Read the model definition and answer for the solid it produces. Units are mm, in the model's axes. A direction names the side the tool comes from. Coordinates: 2 decimals unless noted, no trailing zeros. Order: outer loops, then holes, each group sorted by start corner. A loop starts at its lowest first (then second) coordinate and runs counter-clockwise, first axis right, second up. Notation, with made-up numbers: M -25.5,65 L -3.5,65 A19 ccw -3.5,84 Z; hole C 28,6.25 d11. An arc over 180 degrees is marked long. Use a Markdown table: item, result. Add a question column.
1) Each of these flat-tipped pins is pushed along its axis until it touches: pin 1 Ø3.5 at (x, y) = (8, -20.16) entering from -Z; pin 2 Ø1 at (x, y) = (0.5, -19) entering from +Z; pin 3 Ø4 at (y, z) = (-3.5, 3) entering from -X; pin 4 Ø8 at (y, z) = (-11, 13.5) entering from +X. Where does it stop, or does it pass through?
2) Find section D-D on z = 12.5. Write down the section's boundary in (x, y).
3) Find section C-C on x = -8. Write down the section's boundary in (y, z), plus the area to 3 significant figures.
4) Find the intervals of material crossed by probe 1 along X at (y, z) = (-5, 12.5); probe 2 along Y at (x, z) = (-8, 11.5); probe 3 along X at (y, z) = (-21, 10.25), in increasing order. Write a range as [from, to].
5) Find section B-B on y = -12. Write down the section's boundary in (x, z).
6) For faces 4 (the face through (-0.463, -9.753, 11.864)), 5 (the face through (-2, -10, 23.4)), determine the directions among +Z, -Z, +X, -X, +Y, -Y from which every point of the face is accessible in a straight line to the end or side of a thin tool.
7) The mould has two halves that part along Y. Classify faces 1 (the face through (7.74, -18.175, 12.878)), 2 (the face through (-5.488, -24.713, 12.522)), 3 (the face through (0, 0, 25.4)): released by +Y, released by -Y, zero draft, split by the parting line, or undercut.
8) Find section A-A on x = 0. Write down the section's boundary in (y, z).
from build123d import *

# Parameters (mm, degrees)
SKETCH1_R           = 25.314646171
BOSS_EXTRUDE1_DEPTH = 25.4
SKETCH2_R           = 3.556
CUT_EXTRUDE1_DEPTH  = 25.4
SKETCH3_R           = 7
SKETCH3_R_2         = 3.556
CUT_EXTRUDE2_DEPTH  = 2
SKETCH4_R           = 2
CUT_EXTRUDE3_DEPTH  = 26.4


with BuildPart() as part:
    # Sketch1 → Boss-Extrude1 (new body)
    with BuildSketch(Plane.XY):
        Circle(SKETCH1_R)
    extrude(amount=BOSS_EXTRUDE1_DEPTH)

    # Sketch2 → Cut-Extrude1 (cut)
    with BuildSketch(Plane.XY.offset(25.4)):
        with Locations((0, -13.278788033)):
            Circle(SKETCH2_R)
    extrude(amount=-CUT_EXTRUDE1_DEPTH, mode=Mode.SUBTRACT)

    # Sketch3 → Cut-Extrude2 (cut)
    with BuildSketch(Plane.XY.offset(25.4)):
        with Locations((0, -13.278788033)):
            Circle(SKETCH3_R)
        with Locations((0, -13.278788033)):
            Circle(SKETCH3_R_2, mode=Mode.SUBTRACT)
    extrude(amount=-CUT_EXTRUDE2_DEPTH, mode=Mode.SUBTRACT)

    # Sketch4 → Cut-Extrude3 (cut, through all)
    with BuildSketch(Plane.XY.offset(25.4)):
        with Locations((-8, -4.158160147)):
            Circle(SKETCH4_R)
        with Locations((8, -4.158160147)):
            Circle(SKETCH4_R)
        with Locations((8, -20.158160147)):
            Circle(SKETCH4_R)
        with Locations((-8, -20.158160147)):
            Circle(SKETCH4_R)
    extrude(amount=-CUT_EXTRUDE3_DEPTH, mode=Mode.SUBTRACT)


solid = part.part
Check result:
| question | item | result |
|---|---|---|
| 1 | pin 1 | passes through |
| 1 | pin 2 | stops at z = 23.4 |
| 1 | pin 3 | stops at x = -25.27 |
| 1 | pin 4 | stops at x = 24.33 |
| 2 | outline | C 0,0 d50.63; hole C -8,-20.16 d4; hole C -8,-4.16 d4; hole C 0,-13.28 d7.11; hole C 8,-20.16 d4; hole C 8,-4.16 d4 |
| 3 | outline | M -24.02,0 L -22.16,0 L -22.16,25.4 L -24.02,25.4 Z; M -18.16,0 L -6.16,0 L -6.16,25.4 L -18.16,25.4 Z; M -2.16,0 L 24.02,0 L 24.02,25.4 L -2.16,25.4 Z |
| 3 | area | 1,020 mm2 |
| 4 | probe 1 | x = [-24.82, -9.81], [-6.19, 6.19], [9.81, 24.82] |
| 4 | probe 2 | y = [-24.02, -22.16], [-18.16, -6.16], [-2.16, 24.02] |
| 4 | probe 3 | x = [-14.14, -9.81], [-6.19, 6.19], [9.81, 14.14] |
| 5 | outline | M -22.29,0 L -3.32,0 L -3.32,23.4 L -6.88,23.4 L -6.88,25.4 L -22.29,25.4 Z; M 3.32,0 L 22.29,0 L 22.29,25.4 L 6.88,25.4 L 6.88,23.4 L 3.32,23.4 Z |
| 6 | face 4 | +Z, -Z |
| 6 | face 5 | +Z |
| 7 | face 1 | undercut |
| 7 | face 2 | split by the parting line |
| 7 | face 3 | zero draft |
| 8 | outline | M -25.31,0 L -16.83,0 L -16.83,23.4 L -20.28,23.4 L -20.28,25.4 L -25.31,25.4 Z; M -9.72,0 L 25.31,0 L 25.31,25.4 L -6.28,25.4 L -6.28,23.4 L -9.72,23.4 Z |
